```python
from build123d import *

# Parameters (mm, degrees)
SKETCH_1_R          = 3
EXTRUDE_1_DEPTH     = 105
CUT_EXTRUDE_1_DEPTH = 30
CUT_EXTRUDE_START   = -10
CUT_EXTRUDE_2_DEPTH = 10
M3X0_5_1_D          = 2.5
M3X0_5_1_DEPTH      = 10
M3X0_5_1_TIP        = 0.751075774
CHAMFER_1_SIZE      = 0.5


with BuildPart() as part:
    # 草图1 → 凸台-拉伸1 (new body)
    with BuildSketch(Plane.XY):
        Circle(SKETCH_1_R)
    extrude(amount=EXTRUDE_1_DEPTH)

    # 草图2 → 切除-拉伸1 (cut)
    with BuildSketch(Plane(origin=(0, 0, 0), x_dir=(-1, 0, 0), z_dir=(0, 0, -1))):
        with BuildLine():
            ThreePointArc((3, 0), (2.771638598, 1.148050297), (2.121320344, 2.121320344))
            Line((2.121320344, 2.121320344), (2.121320344, -2.121320344))
            ThreePointArc((2.121320344, -2.121320344), (2.771638598, -1.148050297), (3, 0))
        make_face()
    extrude(amount=-CUT_EXTRUDE_1_DEPTH, mode=Mode.SUBTRACT)

    # 草图3 → 切除-拉伸2 (cut)
    with BuildSketch(Plane.XY.offset(105).offset(CUT_EXTRUDE_START)):
        with BuildLine():
            Line((-2.121320344, -2.121320344), (-2.121320344, 2.121320344))
            ThreePointArc((-2.121320344, 2.121320344), (-3, 0), (-2.121320344, -2.121320344))
        make_face()
    extrude(amount=CUT_EXTRUDE_2_DEPTH, mode=Mode.SUBTRACT)

    # M3x0.5 螺纹孔1
    with Locations(Plane(origin=(0, 0, 0), x_dir=(-1, 0, 0), z_dir=(0, 0, -1))):
        with Locations((0, 0)):
            Hole(M3X0_5_1_D / 2, depth=M3X0_5_1_DEPTH)
            with Locations((0, 0, -(M3X0_5_1_DEPTH + M3X0_5_1_TIP / 2))):  # 118° drill point
                Cone(0, M3X0_5_1_D / 2, M3X0_5_1_TIP, mode=Mode.SUBTRACT)

    # 倒角1
    chamfer_1_edges = [part.edges().sort_by_distance(p)[0] for p in [
        (1.148050297, -2.771638598, 105),
        (-2.121320344, 0, 105),
        (1.148050297, 2.771638598, 0),
        (-2.121320344, 0, 0),
    ]]
    chamfer(chamfer_1_edges, length=CHAMFER_1_SIZE)


solid = part.part
```
Here's how the part is built. I have some questions about the finished solid (model axes, mm). A direction names the side the tool comes from. Round coordinates to 2 decimals unless told otherwise and drop trailing zeros. Order: outer loops, then holes, each group sorted by start corner. A loop starts at its lowest first (then second) coordinate and runs counter-clockwise, first axis right, second up. Notation, with made-up numbers: M 23,6.5 L 73,6.5 A27 cw 73,44.5 Z; hole C -26,-37 d3. An arc over 180 degrees is marked long. One line per question, with ' | ' between items.
1) If we mould it in two halves opening along X, with no side actions, what happens to faces 4 (the face through (0, 0, 105)), 5 (the face through (-2.121, 0, 15)), 6 (the face through (2.634, -0.087, 0.135)), 7 (the face through (0.05, -0.21, 10.62))? For each: +X half, -X half, draft (parallel to the pull), parting line (faces both ways), or undercut.
Working result:
face 4: draft | face 5: -X half | face 6: parting line | face 7: undercut
2) For pin 1 Ø1 at (x, y) = (-2.5, 0) entering from +Z; pin 2 Ø2 at (x, y) = (-1.5, -2) entering from -Z; pin 3 Ø2 at (y, z) = (-1, 100) entering from -X; pin 4 Ø1.5 at (x, y) = (0, 0) entering from -Z, each with a flat end and sliding along its axis, tell me the tip position at first contact or that it passes through.
Working result:
pin 1: z = 104.62 | pin 2: z = 0 | pin 3: x = -2.12 | pin 4: z = 10.3
3) I want a section at A-A, the plane z = 68.5. Write out the boundary of the cut face in (x, y), then the cut area to 3 significant figures.
Working result:
outline: C 0,0 d6 | area: 28.3 mm²
4) I want a section at B-B, the plane z = 12. Write out the boundary of the cut face in (x, y).
Working result:
outline: M -2.12,-2.12 A3 ccw long -2.12,2.12 Z
5) I need wall thicknesses on line 1 along X through (y, z) = (0, 6); line 2 along Y through (x, z) = (0, 4.75); line 3 along Y through (x, z) = (-0.4, 13). Which ranges of each line are inside material? Lowest first, please.
Working result:
line 1: -2.12 to -1.25, 1.25 to 3 | line 2: -3 to -1.25, 1.25 to 3 | line 3: -2.97 to 2.97
6) For faces 1 (the face through (-2.121, 0, 100)), 2 (the face through (2.634, -0.087, 104.865)), 3 (the face through (-0.27, -1.22, 5.07)), which set-ups out of +Z, -Z, +X, -X, +Y, -Y let a thin tool reach every point of the face, with its end or its side?
Working result:
face 1: +Z, -X, +Y, -Y | face 2: +Z | face 3: -Z
